Could you check a few things on this model? Use its own coordinates, in mm. A direction names the side the tool comes from. Give positions to 0.01 mm unless a question says otherwise; leave off trailing zeros. Loops run counter-clockwise (first coordinate to the right, second up) from the corner with the lowest first, then second, coordinate; pieces in that order, holes last. Notation, with made-up numbers: (10, 72.5) - (59, 72.5) arc R28 ccw to (59, 101.5) - close; hole circle Ø4 at (89.5, 7.5). An arc over 180 degrees is marked (long way). One line per item, written item: value. Start each with the question number.
Q1. If we mould it in two halves opening along X, with no side actions, what happens to faces 1 (the face through (-3, 10, 15)), 2 (the face through (-12, 8, 15)), 3 (the face through (-17, 5, 15))? For each: released by +X, released by -X, zero draft, split by the parting line, or undercut.
Q2. I want a section at C-C (x = -9). Please give me the cut outline in (y, z).
Q3. I want a section at B-B (z = 16.75). Please give me the cut outline in (x, y), then the cut area to 3 significant figures.
Q4. I want a section at A-A (y = 9.25). Please give me the cut outline in (x, z).
Q5. For faces 4 (the face through (0, 5, 15)), 5 (the face through (-9, 6, 15)), which set-ups out of +Z, -Z, +X, -X, +Y, -Y let a thin tool reach every point of the face, with its end or its side?
Q6. If I drill on line 1 (X direction, y = 7.75, z = 9.5); line 2 (Y direction, x = -6.75, z = 28.5), over which ranges is the centre line in solid material (lowest first)? Write a range as from..to.
Autodesk Inventor part; units mm, degrees
ref_plane "YZ Plane" through (0, 0, 0) normal (1, 0, 0) x (0, 1, 0)
ref_plane "XZ Plane" through (0, 0, 0) normal (0, 1, 0) x (-1, 0, 0)
ref_plane "XY Plane" through (0, 0, 0) normal (0, 0, 1) x (1, 0, 0)
sketch "Sketch1" plane through (0, 0, 0) normal (0, 0, 1) x (1, 0, 0)
  line L0 (0, 0) -> (-17, 0)
  line L1 (-17, 0) -> (-17, 10)
  line L2 (-17, 10) -> (0, 10)
  line L3 (0, 10) -> (0, 0)
  line L4 (-5, 10) -> (-12, 10)
  line L5 (-12, 10) -> (-12, 6)
  line L6 (-12, 6) -> (-5, 6)
  line L7 (-5, 6) -> (-5, 10)
  dimension "d0" = 17
  dimension "d2" = 4
  dimension "d3" = 7
  dimension "d4" = 5
  dimension "d5" = 6
extrude "Extrusion1" add sketch "Sketch1" along normal blind 30 contours L0 L1 L2 L5 L6 L7 L3
properties part number "Top Rack V2"
Worked answers:
1. face 1: zero draft
1. face 2: undercut
1. face 3: released by -X
2. outline: (0, 0) - (6, 0) - (6, 30) - (0, 30) - close
3. outline: (-17, 0) - (0, 0) - (0, 10) - (-5, 10) - (-5, 6) - (-12, 6) - (-12, 10) - (-17, 10) - close
3. area: 142 mm²
4. outline: (-17, 0) - (-12, 0) - (-12, 30) - (-17, 30) - close; (-5, 0) - (0, 0) - (0, 30) - (-5, 30) - close
5. face 4: +Z, -Z, +X, +Y, -Y
5. face 5: +Z, -Z, +Y
6. line 1: x = -17..-12, -5..0
6. line 2: y = 0..6
